```python
from build123d import *

# Parameters (mm, degrees)
SKETCH1_R                 = 11
SKETCH1_R_2               = 4.1
BOSS_EXTRUDE1_DEPTH       = 2
M2X0_4_TAPPED_HOLE1_D     = 1.6
M2X0_4_TAPPED_HOLE1_DEPTH = 5.2
M2X0_4_TAPPED_HOLE1_TIP   = 0.480688495
SKETCH5_R                 = 5
SKETCH5_R_2               = 4.1
BOSS_EXTRUDE2_DEPTH       = 1


with BuildPart() as part:
    # Sketch1 → Boss-Extrude1 (new body)
    with BuildSketch(Plane.XY):
        Circle(SKETCH1_R)
        Circle(SKETCH1_R_2, mode=Mode.SUBTRACT)
    extrude(amount=BOSS_EXTRUDE1_DEPTH)

    # M2x0.4 Tapped Hole1
    with Locations(Plane.XY.offset(2)):
        with Locations((0, 8), (5.656854249, 5.656854249), (8, 0), (5.656854249, -5.656854249), (0, -8), (-5.656854249, -5.656854249), (-8, 0), (-5.656854249, 5.656854249)):
            Hole(M2X0_4_TAPPED_HOLE1_D / 2, depth=M2X0_4_TAPPED_HOLE1_DEPTH)
            with Locations((0, 0, -(M2X0_4_TAPPED_HOLE1_DEPTH + M2X0_4_TAPPED_HOLE1_TIP / 2))):  # 118° drill point
                Cone(0, M2X0_4_TAPPED_HOLE1_D / 2, M2X0_4_TAPPED_HOLE1_TIP, mode=Mode.SUBTRACT)

    # Sketch5 → Boss-Extrude2 (add)
    with BuildSketch(Plane.XY.offset(2)):
        Circle(SKETCH5_R)
        Circle(SKETCH5_R_2, mode=Mode.SUBTRACT)
    extrude(amount=BOSS_EXTRUDE2_DEPTH)


solid = part.part
```
Geometry check sheet. Reference: the model listing, model coordinates, mm. A direction names the side the tool comes from. Round coordinates to 2 decimals unless told otherwise and drop trailing zeros. Order: outer loops, then holes, each group sorted by start corner. A loop starts at its lowest first (then second) coordinate and runs counter-clockwise, first axis right, second up. Notation, with made-up numbers: (-19, -9) - (-9, -9) arc R25 cw to (-9, 19) - close; hole circle Ø1 at (82.5, 22.5). An arc over 180 degrees is marked (long way). Use a Markdown table: item, result. Add a question column.
(1) Tool access check on faces 4 (the cylindrical face through (-2.38, -10.74, 0.99)), 5 (the flat face through (5, -2, 2)). Record the directions out of +Z, -Z, +X, -X, +Y, -Y that give a thin tool (end or side, any length) a straight path to the whole face; none if there is none.
(2) Depth check by flat-ended pin: pin 1 (1.8 mm diameter, centred on x = -5.66, y = 5.66, fed in from +Z). Enter the tip coordinate at first touch or a pass-through.
(3) Sectioned sample at C-C, the plane y = 3. Enter the section's corners in (x, z), and give its area (3 significant figures).
(4) Sectioned sample at A-A, the plane y = 0. Enter the section's corners in (x, z).
(5) Material ranges on line 1 along Y through (x, z) = (0, 0.95); line 2 along Z through (x, y) = (4.5, 7.25); line 3 along X through (y, z) = (5.5, 1.8), recorded low to high. Write a range as [from, to].
(6) Sectioned sample at D-D, the plane z = 1.35. Count the separate pieces of the cut face and the enclosed holes in it, and give its area (3 significant figures).
(7) Release check for a two-part mould opening along X. For faces 1 (the flat face through (0, -5, 0)), 2 (the cylindrical face through (-1.08, -4.88, 2.49)), 3 (the cylindrical face through (-0.534, 4.065, 1.479)) record: pulls with the +X half, pulls with the -X half, needs draft (parallel to the pull), parting line crosses it, or undercut.
Answers below:
| question | item | result |
|---|---|---|
| 1 | face 4 | +Z, -Z |
| 1 | face 5 | +Z |
| 2 | pin 1 | z = 2 |
| 3 | outline | (-10.58, 0) - (-2.79, 0) - (-2.79, 3) - (-4, 3) - (-4, 2) - (-10.58, 2) - close; (2.79, 0) - (10.58, 0) - (10.58, 2) - (4, 2) - (4, 3) - (2.79, 3) - close |
| 3 | area | 33.6 mm² |
| 4 | outline | (-11, 0) - (-8.8, 0) - (-8.8, 2) - (-11, 2) - close; (-7.2, 0) - (-4.1, 0) - (-4.1, 3) - (-5, 3) - (-5, 2) - (-7.2, 2) - close; (4.1, 0) - (7.2, 0) - (7.2, 2) - (5, 2) - (5, 3) - (4.1, 3) - close; (8.8, 0) - (11, 0) - (11, 2) - (8.8, 2) - close |
| 5 | line 1 | [-11, -8.8], [-7.2, -4.1], [4.1, 7.2], [8.8, 11] |
| 5 | line 2 | [0, 2] |
| 5 | line 3 | [-9.53, -6.44], [-4.87, 4.87], [6.44, 9.53] |
| 6 | separate pieces | 1 |
| 6 | enclosed holes | 9 |
| 6 | area | 311 mm² |
| 7 | face 1 | needs draft |
| 7 | face 2 | parting line crosses it |
| 7 | face 3 | undercut |
